Could you check a few things on this model? Use its own coordinates, in mm. A direction names the side the tool comes from. Coordinates: 2 decimals unless noted, no trailing zeros. Write each loop counter-clockwise with the first axis right and the second up, starting at its lowest first coordinate (ties: lowest second). Pieces come first, ordered by that corner, then holes.
Item 1: I want a section at D-D on z = 9. Please give me the cut outline in (x, y), then the cut area to 3 significant figures.
Item 2: Thinking about a two-plate mould opening in X: for faces 1 (the cylindrical face through (-62.91, 12.36, 32.31)), 2 (the flat face through (55, 10, 2)), 3 (the flat face through (7.3, 7, 43.2)), which applies, +X half, -X half, draft (parallel to the pull), parting line (faces both ways), or undercut?
Item 3: I want a section at B-B on y = 17.5. Please give me the cut outline in (x, z).
Item 4: I want a section at C-C on x = 0. Please give me the cut outline in (y, z), then the cut area to 3 significant figures.
Item 5: For P1, Ø1.5, axis at y = 12.5, z = 33.5, coming from the +X side; P2, Ø1, axis at y = 15, z = 16, coming from the +X side; P3, Ø4, axis at y = 5, z = 29, coming from the -X side, each with a flat end and sliding along its axis, tell me the tip position at first contact or that it passes through.
Item 6: If I drill on probe 1 along X at (y, z) = (10, 12.5); probe 2 along X at (y, z) = (10, 18.5); probe 3 along Z at (x, y) = (-39, 13.75), over which ranges is the centre line in solid material (lowest first)?
Item 7: I want a section at A-A on z = 19. Please give me the cut outline in (x, y).
Item 8: Which directions (+Z, -Z, +X, -X, +Y, -Y) give clear straight access to the entire face, cutting with the end or side of a thin tool? Please do faces 4 (the cylindrical face through (63.104, 8.698, 12.321)), 5 (the cylindrical face through (-1.02, 13.59, 47.49)), 6 (the cylindrical face through (-0.93, 3.45, 43.49)).
from build123d import *

# Parameters (mm, degrees)
SKETCH1_R                   = 62.5
SKETCH1_R_2                 = 43.5
BOSS_EXTRUDE1_DEPTH         = 20
SKETCH2_R                   = 47.5
CUT_EXTRUDE1_DEPTH          = 13
SKETCH3_R                   = 4
CUT_EXTRUDE2_DEPTH          = 91.622844802
SKETCH4_W                   = 150
SKETCH4_H                   = 64.5
SKETCH4_W_2                 = 72.256487598
SKETCH4_H_2                 = 11.5
CUT_EXTRUDE3_DEPTH          = 91.622844802
BOSS_EXTRUDE4_DEPTH         = 20
SKETCH7_R                   = 2.5
CUT_EXTRUDE4_DEPTH          = 90.742875716
M8_TAPPED_HOLE1_D           = 6.8
M8_TAPPED_HOLE1_DEPTH       = 38.75
M8_TAPPED_HOLE1_CSINK_D     = 8.05
M8_TAPPED_HOLE1_CSINK_ANGLE = 90
M8_TAPPED_HOLE1_TIP         = 2.042926105
M8_TAPPED_HOLE2_D           = 6.8
M8_TAPPED_HOLE2_DEPTH       = 19.75
M8_TAPPED_HOLE2_CSINK_D     = 8.05
M8_TAPPED_HOLE2_CSINK_ANGLE = 90
M8_TAPPED_HOLE2_TIP         = 2.042926105


with BuildPart() as part:
    # Sketch1 → Boss-Extrude1 (new body)
    with BuildSketch(Plane(origin=(0, 0, 0), x_dir=(1, 0, 0), z_dir=(0, 1, 0))):
        with Locations(Location((0, 0, 0), (0, 0, 270))):
            Circle(SKETCH1_R)
        with Locations(Location((0, 0, 0), (0, 0, 270))):
            Circle(SKETCH1_R_2, mode=Mode.SUBTRACT)
    extrude(amount=BOSS_EXTRUDE1_DEPTH)

    # Sketch2 → Cut-Extrude1 (cut)
    with BuildSketch(Plane(origin=(0, 20, 0), x_dir=(1, 0, 0), z_dir=(0, 1, 0))):
        with Locations(Location((0, 0, 0), (0, 0, 270))):
            Circle(SKETCH2_R)
    extrude(amount=-CUT_EXTRUDE1_DEPTH, mode=Mode.SUBTRACT)

    # Sketch3 → Cut-Extrude2 (cut, through all)
    with BuildSketch(Plane(origin=(0, 20, 0), x_dir=(1, 0, 0), z_dir=(0, 1, 0))):
        with Locations(Location((38.183766184, 38.183766184, 0), (0, 0, 270))):
            Circle(SKETCH3_R)
        with Locations(Location((38.183766184, -38.183766184, 0), (0, 0, 270))):
            Circle(SKETCH3_R)
        with Locations(Location((-38.183766184, -38.183766184, 0), (0, 0, 270))):
            Circle(SKETCH3_R)
        with Locations(Location((-38.183766184, 38.183766184, 0), (0, 0, 270))):
            Circle(SKETCH3_R)
    extrude(amount=-CUT_EXTRUDE2_DEPTH, mode=Mode.SUBTRACT)

    # Sketch4 → Cut-Extrude3 (cut, through all)
    with BuildSketch(Plane(origin=(0, 20, 0), x_dir=(1, 0, 0), z_dir=(0, 1, 0))):
        with Locations((0, 30.25)):
            Rectangle(SKETCH4_W, SKETCH4_H)
        with Locations((0, -56.75)):
            Rectangle(SKETCH4_W_2, SKETCH4_H_2)
    extrude(amount=-CUT_EXTRUDE3_DEPTH, mode=Mode.SUBTRACT)

    # Sketch6 → Boss-Extrude4 (add, through all)
    with BuildSketch(Plane(origin=(0, 20, 0), x_dir=(1, 0, 0), z_dir=(0, 1, 0))):
        with BuildLine():
            Line((-62.467991804, -2), (-72.467991804, -2))
            ThreePointArc((-72.467991804, -2), (-62.636910051, -32.684277735), (-36.128243799, -51))
            ThreePointArc((-36.128243799, -51), (-55.050471558, -29.592154049), (-62.467991804, -2))
        make_face()
        with BuildLine():
            ThreePointArc((62.467991804, -2), (55.050471558, -29.592154049), (36.128243799, -51))
            ThreePointArc((36.128243799, -51), (62.636910051, -32.684277735), (72.467991804, -2))
            Line((72.467991804, -2), (62.467991804, -2))
        make_face()
    extrude(amount=-BOSS_EXTRUDE4_DEPTH)

    # Sketch7 → Cut-Extrude4 (cut, through all)
    with BuildSketch(Plane(origin=(0, 0, 2), x_dir=(-1, 0, 0), z_dir=(0, 0, -1))):
        with Locations((-59.962933931, 10)):
            Circle(SKETCH7_R)
    extrude(amount=-CUT_EXTRUDE4_DEPTH, mode=Mode.SUBTRACT)

    # M8 Tapped Hole1
    with Locations(Plane(origin=(-59.962933931, 10, 2), x_dir=(-1, 0, 0), z_dir=(0, 0, -1))):
        with Locations((0, 0)):
            CounterSinkHole(M8_TAPPED_HOLE1_D / 2, M8_TAPPED_HOLE1_CSINK_D / 2, depth=M8_TAPPED_HOLE1_DEPTH, counter_sink_angle=M8_TAPPED_HOLE1_CSINK_ANGLE)
            with Locations((0, 0, -(M8_TAPPED_HOLE1_DEPTH + M8_TAPPED_HOLE1_TIP / 2))):  # 118° drill point
                Cone(0, M8_TAPPED_HOLE1_D / 2, M8_TAPPED_HOLE1_TIP, mode=Mode.SUBTRACT)

    # M8 Tapped Hole2
    with Locations(Plane(origin=(59.962933931, 10, 2), x_dir=(-1, 0, 0), z_dir=(0, 0, -1))):
        with Locations((0, 0)):
            CounterSinkHole(M8_TAPPED_HOLE2_D / 2, M8_TAPPED_HOLE2_CSINK_D / 2, depth=M8_TAPPED_HOLE2_DEPTH, counter_sink_angle=M8_TAPPED_HOLE2_CSINK_ANGLE)
            with Locations((0, 0, -(M8_TAPPED_HOLE2_DEPTH + M8_TAPPED_HOLE2_TIP / 2))):  # 118° drill point
                Cone(0, M8_TAPPED_HOLE2_D / 2, M8_TAPPED_HOLE2_TIP, mode=Mode.SUBTRACT)


solid = part.part
Response values:
1. outline: (-72.1, 0) - (-42.56, 0) - (-42.56, 7) - (-46.64, 7) - (-46.64, 20) - (-72.1, 20) - close; (42.56, 0) - (72.1, 0) - (72.1, 20) - (46.64, 20) - (46.64, 7) - (42.56, 7) - close; hole circle Ø6.8 at (-59.96, 10); hole circle Ø6.8 at (59.96, 10)
1. area: 1,000 mm2
2. face 1: -X half
2. face 2: draft
2. face 3: undercut
3. outline: (-72.47, 2) - (-47.46, 2) arc R47.5 cw to (47.46, 2) - (72.47, 2) arc R50 ccw to (36.13, 51) - (-36.13, 51) arc R50 ccw to start; hole circle Ø8 at (-38.18, 38.18); hole circle Ø8 at (38.18, 38.18)
4. outline: (0, 43.5) - (7, 43.5) - (7, 47.5) - (20, 47.5) - (20, 51) - (0, 51) - close
4. area: 98.0 mm2
5. P1: stops at x = 62.59
5. P2: stops at x = 70.86
5. P3: stops at x = -66.28
6. probe 1: x = -71.55 to -63.36, -56.56 to -45.83, 45.83 to 56.56, 63.36 to 71.55
6. probe 2: x = -69.98 to -63.36, -56.56 to -43.75, 43.75 to 56.56, 63.36 to 69.98
6. probe 3: z = 27.12 to 34.27, 42.1 to 50.09
7. outline: (-69.81, 0) - (-39.13, 0) - (-39.13, 7) - (-43.53, 7) - (-43.53, 20) - (-69.81, 20) - close; (39.13, 0) - (69.81, 0) - (69.81, 20) - (43.53, 20) - (43.53, 7) - (39.13, 7) - close; hole circle Ø6.8 at (-59.96, 10); hole circle Ø6.8 at (59.96, 10)
8. face 4: -Z
8. face 5: -Z, +Y
8. face 6: -Z, +Y, -Y
